Geometry: final body of the model. Coordinates: model frame, mm. A direction names the side the tool comes from. Coordinates: 2 decimals unless noted, no trailing zeros. Loops run counter-clockwise (first coordinate to the right, second up) from the corner with the lowest first, then second, coordinate; pieces in that order, holes last. Notation, with made-up numbers: M -39,66.5 L 17,66.5 A21 cw 17,87.5 Z; hole C 21.25,-28 d10. An arc over 180 degrees is marked long. Write item = value, one per line. Start each with the question number.
```python
from build123d import *

# Parameters (mm, degrees)
ESQUISSE1_W             = 159
ESQUISSE1_H             = 40
BOSS_EXTRU_1_DEPTH      = 2
ESQUISSE2_W             = 159
ESQUISSE2_H             = 40
ESQUISSE2_W_2           = 151
ESQUISSE2_H_2           = 37
BOSS_EXTRU_2_DEPTH      = 150
ESQUISSE3_W             = 51
ESQUISSE3_H             = 9.75
ESQUISSE3_H_2           = 13.5
ENL_V_MAT_EXTRU_1_DEPTH = 3


with BuildPart() as part:
    # Esquisse1 → Boss.-Extru.1 (new body)
    with BuildSketch(Plane.XY):
        with Locations((79.5, 20)):
            Rectangle(ESQUISSE1_W, ESQUISSE1_H)
    extrude(amount=BOSS_EXTRU_1_DEPTH)

    # Esquisse2 → Boss.-Extru.2 (add)
    with BuildSketch(Plane.XY.offset(2)):
        with Locations((79.5, 20)):
            Rectangle(ESQUISSE2_W, ESQUISSE2_H)
        with Locations((79.5, 20)):
            Rectangle(ESQUISSE2_W_2, ESQUISSE2_H_2, mode=Mode.SUBTRACT)
    extrude(amount=BOSS_EXTRU_2_DEPTH)

    # Esquisse3 → Enlèv. mat.-Extru.1 (cut)
    with BuildSketch(Plane.ZY):
        with Locations((126.5, 35.125)):
            Rectangle(ESQUISSE3_W, ESQUISSE3_H)
        with Locations((126.5, 20)):
            Rectangle(ESQUISSE3_W, ESQUISSE3_H_2)
        with Locations((126.5, 4.875)):
            Rectangle(ESQUISSE3_W, ESQUISSE3_H)
    extrude(amount=-ENL_V_MAT_EXTRU_1_DEPTH, mode=Mode.SUBTRACT)


solid = part.part
```
Item 1: Line query: line 1 (X direction, y = 19, z = 133.5); line 2 (X direction, y = 29.5, z = 70); line 3 (Y direction, x = 65.5, z = 58). Output: solid intervals per line, ascending. Write a range as from..to.
Item 2: Pull-direction query (Y, two-part tool) for faces 5 (the flat face through (78, 40, 75)), 6 (the flat face through (78, 38.5, 76)), 7 (the flat face through (78, 20, 0)), 8 (the flat face through (78, 0, 75)); classes: released by +Y, released by -Y, zero draft, split by the parting line, or undercut.
Item 3: Section query D-D (z = 107.5). Return the cut outline in (x, y).
Item 4: First-contact query: pin 1 (2.5 mm diameter, centred on x = 1, z = 131.5, fed in from -Y); pin 2 (0.9 mm diameter, centred on x = 1, y = 37, fed in from +Z); pin 3 (8 mm diameter, centred on y = 22.5, z = 122.5, fed in from -X). Flat tips, straight axial feed; report the tip coordinate or a pass-through.
Item 5: Reachability of faces 1 (the flat face through (4, 20, 76)), 2 (the flat face through (3, 5, 126)), 3 (the flat face through (3, 35, 126)), 4 (the flat face through (3, 20, 126)) from +Z, -Z, +X, -X, +Y, -Y: full face, straight path, thin tool, end or side. Return the list, or none.
Item 6: Section query B-B (y = 23). Return the cut outline in (x, z).
Item 7: Section query A-A (z = 17). Return the cut outline in (x, y).
Item 8: Section query C-C (x = 60). Return the cut outline in (y, z).
Verdict:
q1.line_1 = 3..4, 155..159
q1.line_2 = 0..4, 155..159
q1.line_3 = 0..1.5, 38.5..40
q2.face_5 = released by +Y
q2.face_6 = undercut
q2.face_7 = zero draft
q2.face_8 = released by -Y
q3.outline = M 0,9.75 L 3,9.75 L 3,0 L 159,0 L 159,40 L 3,40 L 3,30.25 L 0,30.25 L 0,26.75 L 3,26.75 L 3,13.25 L 0,13.25 Z; hole M 4,1.5 L 155,1.5 L 155,38.5 L 4,38.5 Z
q4.pin_1 = 9.75
q4.pin_2 = 101
q4.pin_3 = 3
q5.face_1 = +Z
q5.face_2 = +Z, -X, -Y
q5.face_3 = +Z, -X, +Y
q5.face_4 = +Z, -X
q6.outline = M 0,0 L 159,0 L 159,152 L 155,152 L 155,2 L 4,2 L 4,152 L 3,152 L 3,101 L 0,101 Z
q7.outline = M 0,0 L 159,0 L 159,40 L 0,40 Z; hole M 4,1.5 L 155,1.5 L 155,38.5 L 4,38.5 Z
q8.outline = M 0,0 L 40,0 L 40,152 L 38.5,152 L 38.5,2 L 1.5,2 L 1.5,152 L 0,152 Z
